Verification items for the finished model (mm, model axes). Give positions to 0.01 mm unless a question says otherwise; leave off trailing zeros. Order: outer loops, then holes, each group sorted by start corner. A loop starts at its lowest first (then second) coordinate and runs counter-clockwise, first axis right, second up.
(1) Sectioned sample at B-B on y = -0.5. Record the cut outline in (x, z) (3 decimals).
(2) Scan lines: L1, parallel to Y at x = 0, z = 40 (3 decimals); L2, parallel to Y at x = 0, z = 6.5 (3 decimals); L3, parallel to Z at x = -0.25, y = 0.25. Record each from-to range of solid material in increasing order.
(3) Sectioned sample at A-A on x = 0. Record the cut outline in (y, z) (3 decimals), plus the area to 3 significant figures.
(4) Sectioned sample at D-D on x = 2.5. Record the cut outline in (y, z) (3 decimals), plus the area to 3 significant figures.
(5) Sectioned sample at C-C on z = 26. Record the cut outline in (x, y) (3 decimals).
(6) Gauge pin test, flat ends, axial feed: pin 1 (0.9 mm diameter, centred on x = 0, y = 0, fed in from -Z); pin 2 (4 mm diameter, centred on x = 1.5, y = -1, fed in from -Z). Record the tip position at first contact, or that the pin passes through.
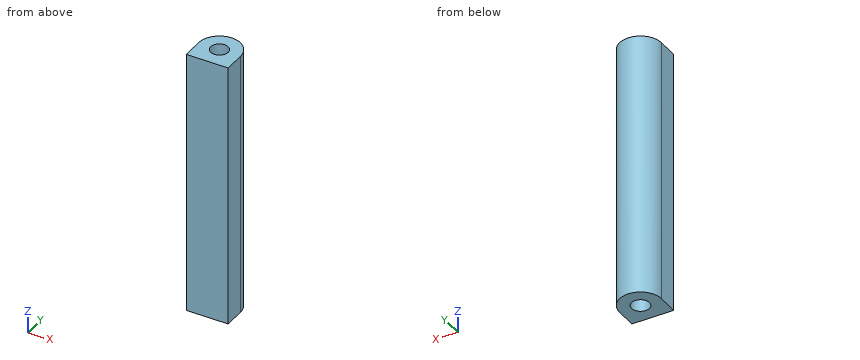
```python
from build123d import *

# Parameters (mm, degrees)
SKETCH1_R           = 3.425
BOSS_EXTRUDE1_DEPTH = 43.5096
SKETCH2_R           = 1.475
CUT_EXTRUDE1_DEPTH  = 10
SKETCH3_R           = 1.425
CUT_EXTRUDE2_DEPTH  = 10
BOSS_EXTRUDE2_START = -43.5096
BOSS_EXTRUDE2_DEPTH = 43.5096


with BuildPart() as part:
    # Sketch1 → Boss-Extrude1 (new body)
    with BuildSketch(Plane.XY):
        Circle(SKETCH1_R)
    extrude(amount=BOSS_EXTRUDE1_DEPTH)

    # Sketch2 → Cut-Extrude1 (cut)
    with BuildSketch(Plane(origin=(0, 0, 0), x_dir=(-1, 0, 0), z_dir=(0, 0, -1))):
        Circle(SKETCH2_R)
    extrude(amount=-CUT_EXTRUDE1_DEPTH, mode=Mode.SUBTRACT)

    # Sketch3 → Cut-Extrude2 (cut)
    with BuildSketch(Plane.XY.offset(43.5096)):
        Circle(SKETCH3_R)
    extrude(amount=-CUT_EXTRUDE2_DEPTH, mode=Mode.SUBTRACT)

    # Sketch4 → Boss-Extrude2 (add)
    with BuildSketch(Plane.XY.offset(43.5096).offset(BOSS_EXTRUDE2_START)):
        with BuildLine():
            Line((-3.425, -3.425), (0, -3.425))
            ThreePointArc((0, -3.425), (-2.421840726, -2.421840726), (-3.425, 0))
            Line((-3.425, 0), (-3.425, -3.425))
        make_face()
        with BuildLine():
            ThreePointArc((3.425, 0), (2.421840726, -2.421840726), (0, -3.425))
            Line((0, -3.425), (1.146126532, -3.425))
            Line((1.146126532, -3.425), (3.425, -3.425))
            Line((3.425, -3.425), (3.425, 0))
        make_face()
    extrude(amount=BOSS_EXTRUDE2_DEPTH)


solid = part.part
```
Ans:
1. outline: (-3.425, 0) - (-1.388, 0) - (-1.388, 10) - (1.388, 10) - (1.388, 0) - (3.425, 0) - (3.425, 43.51) - (1.334, 43.51) - (1.334, 33.51) - (-1.334, 33.51) - (-1.334, 43.51) - (-3.425, 43.51) - close
2. L1: y = -3.425 to -1.425, 1.425 to 3.425
2. L2: y = -3.425 to -1.475, 1.475 to 3.425
2. L3: z = 10 to 33.51
3. outline: (-3.425, 0) - (-1.475, 0) - (-1.475, 10) - (1.475, 10) - (1.475, 0) - (3.425, 0) - (3.425, 43.51) - (1.425, 43.51) - (1.425, 33.51) - (-1.425, 33.51) - (-1.425, 43.51) - (-3.425, 43.51) - close
3. area: 240 mm2
4. outline: (-3.425, 0) - (2.341, 0) - (2.341, 43.51) - (-3.425, 43.51) - close
4. area: 251 mm2
5. outline: (-3.425, -3.425) - (3.425, -3.425) - (3.425, 0) arc R3.425 ccw to (-3.425, 0) - close
6. pin 1: stops at z = 10
6. pin 2: stops at z = 0
